from build123d import *

# Parameters (mm, degrees)
BOSS_EXTRU_1_DEPTH      = 472
ESQUISSE2_W             = 165
ESQUISSE2_H             = 124
ENL_V_MAT_EXTRU_1_DEPTH = 22
ESQUISSE3_W             = 50
ESQUISSE3_H             = 22
ENL_V_MAT_EXTRU_2_DEPTH = 70
ENL_V_MAT_EXTRU_3_DEPTH = 120


with BuildPart() as part:
    # Esquisse1 → Boss.-Extru.1 (new body)
    with BuildSketch(Plane.XY):
        with BuildLine():
            Line((-11, -38.457769046), (-11, -84))
            Line((-11, -84), (11, -84))
            Line((11, -84), (11, -38.457769046))
            ThreePointArc((11, -38.457769046), (38.722583559, -10.028036822), (28.284271247, 28.284271247))
            Line((28.284271247, 28.284271247), (26.870057685, 26.870057685))
            ThreePointArc((26.870057685, 26.870057685), (0, -38), (-26.870057685, 26.870057685))
            Line((-26.870057685, 26.870057685), (-28.284271247, 28.284271247))
            ThreePointArc((-28.284271247, 28.284271247), (-38.722583559, -10.028036822), (-11, -38.457769046))
        make_face()
    extrude(amount=BOSS_EXTRU_1_DEPTH)

    # Esquisse2 → Enlèv. mat.-Extru.1 (cut)
    with BuildSketch(Plane.XY.offset(472)):
        Rectangle(ESQUISSE2_W, ESQUISSE2_H)
    extrude(amount=-ENL_V_MAT_EXTRU_1_DEPTH, mode=Mode.SUBTRACT)

    # Esquisse3 → Enlèv. mat.-Extru.2 (cut)
    with BuildSketch(Plane.XY.offset(450)):
        with Locations((0, -51)):
            Rectangle(ESQUISSE3_W, ESQUISSE3_H)
    extrude(amount=-ENL_V_MAT_EXTRU_2_DEPTH, mode=Mode.SUBTRACT)

    # Esquisse4 → Enlèv. mat.-Extru.3 (cut)
    with BuildSketch(Plane.XY.offset(450)):
        Polygon((-67.5, 20), (-67.5, -20), (67.5, -20), (67.5, 20), (67.5, 60), (-67.5, 60), align=None)
    extrude(amount=-ENL_V_MAT_EXTRU_3_DEPTH, mode=Mode.SUBTRACT)

    # Esquisse6 → Révolution1 (revolve)
    with BuildSketch(Plane(origin=(0, 0, 0), x_dir=(1, 0, 0), z_dir=(0, 1, 0)), mode=Mode.PRIVATE) as r_volution1_sk:
        Polygon((0, 80), (-40, 0), (-38, 0), (0, 76), align=None)
    revolve(r_volution1_sk.sketch.rotate(Axis((0, 0, 0), (0, 0, -1)), 180), axis=Axis((0, 0, 0), (0, 0, -1)))


solid = part.part
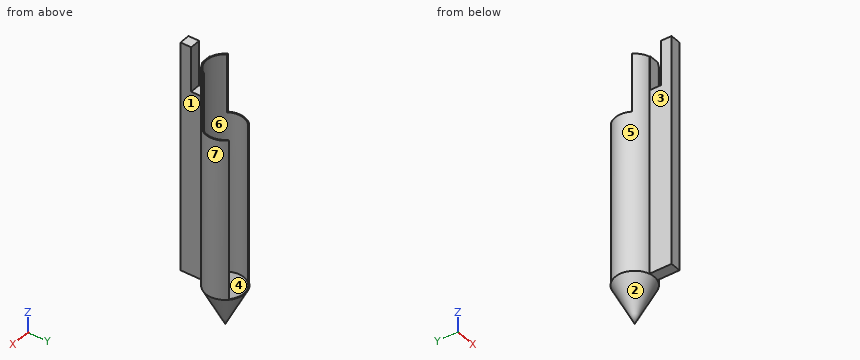
Build history of the part. All positions in model axes, mm. Face numbers are marked on the shaded views. A direction names the side the tool comes from. Round coordinates to 2 decimals unless told otherwise and drop trailing zeros. Loops run counter-clockwise (first coordinate to the right, second up) from the corner with the lowest first, then second, coordinate; pieces in that order, holes last. Notation, with made-up numbers: (71.5, -25) -> (108.5, -25) arc R22 ccw to (108.5, -10) -> close; hole circle Ø11 at (82.5, -20.5). An arc over 180 degrees is marked (long way). One line per item, written item: value. Start each with the question number.
Q1. 3-axis set-ups, long thin cutter, end or side, ignore diameter. For the marked faces 1, 2 and 3: which of +Z, -Z, +X, -X, +Y, -Y reach the whole face in a straight line?
Q2. Probe line 1 along X through (y, z) = (0, 123); line 2 along Y through (x, z) = (0, 333); line 3 along Z through (x, y) = (-5, -48). List the from-to ranges inside material, lowest first.
Q3. Two-plate mould, pull along X, no slides. Class the marked faces 4, 5, 6 and 7: released by +X, released by -X, zero draft, split by the parting line, or undercut.
Q4. Cut at B-B on z = 291. List the corners of the cut face in (x, y), plus the area to 3 significant figures.
Q5. Cut at A-A on z = 349. List the corners of the cut face in (x, y).
Q6. Drop flat-ended pins along their axis: pin 1 Ø2 at (x, z) = (23, 197.5) entering from -Y; pin 2 Ø6 at (x, y) = (13.5, -14.5) entering from -Z; pin 3 Ø23 at (y, z) = (-53, 243.5) entering from -X. Give the stop position or say it passes through.
Computed:
1. face 1: +Z, -Z, +X, -Y
1. face 2: -Z
1. face 3: +Z, -Z, -X, -Y
2. line 1: -40 to -38, 38 to 40
2. line 2: -84 to -38
2. line 3: 0 to 380
3. face 4: undercut
3. face 5: released by -X
3. face 6: undercut
3. face 7: released by +X
4. outline: (-28.28, 28.28) arc R40 ccw to (-11, -38.46) -> (-11, -84) -> (11, -84) -> (11, -38.46) arc R40 ccw to (28.28, 28.28) -> (26.87, 26.87) arc R38 cw (long way) to (-26.87, 26.87) -> close
4. area: 1,350 mm²
5. outline: (-34.64, -20) arc R40 ccw to (-11, -38.46) -> (-11, -84) -> (11, -84) -> (11, -38.46) arc R40 ccw to (34.64, -20) -> (32.31, -20) arc R38 cw to (-32.31, -20) -> close
6. pin 1: y = -33.41
6. pin 2: z = -46.38
6. pin 3: x = -11
